CAD build for the part. Positions are in the model's coordinates, mm. Face numbers are marked on the shaded views. A direction names the side the tool comes from. Coordinates: 2 decimals unless noted, no trailing zeros. Order: outer loops, then holes, each group sorted by start corner. A loop starts at its lowest first (then second) coordinate and runs counter-clockwise, first axis right, second up. Notation, with made-up numbers: (51.5, -31.5) - (93.5, -31.5) arc R10 cw to (93.5, -22.5) - close; hole circle Ø8 at (84.5, 28). An arc over 180 degrees is marked (long way). Write each question's results on one line, items separated by ' | '. Start each with the question number.
Q1. Wall check: probe 1 along X at (y, z) = (-1.5, 19.25); probe 2 along Y at (x, z) = (-15.9, 10); probe 3 along Y at (x, z) = (-17, 12.5). Give the ranges that are in metal, low to high.
Q2. Pin check, flat tips, straight feed: P1, Ø12, axis at x = -12, z = 6.5, coming from the +Y side; P2, Ø5, axis at x = -0.63, z = 10, coming from the +Y side. Stop position of each tip, or through.
Q3. Band-saw the part on B-B, the plane y = 8. Write the cut outline in (x, z), then the cut area to 3 significant figures.
Q4. Band-saw the part on C-C, the plane z = 10. Count the separate pieces of the cut face and the enclosed holes in it, then the cut area to 3 significant figures.
Q5. Band-saw the part on D-D, the plane x = -3. Write the cut outline in (y, z), then the cut area to 3 significant figures.
Q6. Band-saw the part on A-A, the plane y = -6.5. Write the cut outline in (x, z), then the cut area to 3 significant figures.
Q7. Pull direction X, two halves, no side cores. Call the marked faces 3, 4 and 5: released by +X, released by -X, zero draft, split by the parting line, or undercut.
Q8. Which spindle directions (+Z, -Z, +X, -X, +Y, -Y) get a long thin tool onto all of the face, cutting with end or side? Do the marked faces 1 and 2. Say none if no direction does.
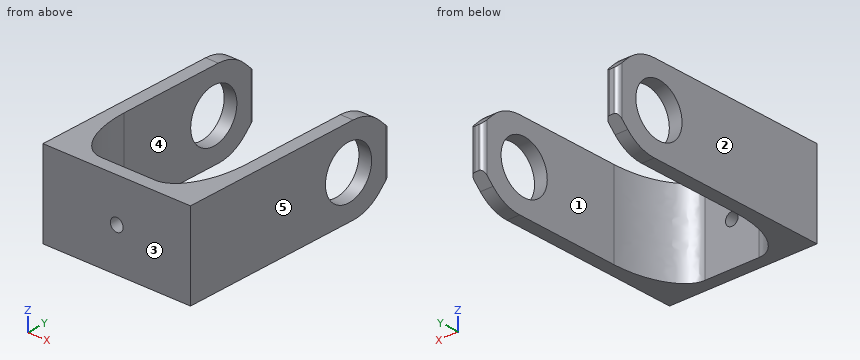
```python
from build123d import *

# Parameters (mm, degrees)
EXTRUDE_1_DEPTH     = 20
CUT_EXTRUDE_1_REACH = 52.828
SKETCH_2_R          = 6.1
SKETCH_3_R          = 1.5
CUT_EXTRUDE_2_DEPTH = 52.5
FILLET_1_R          = 10
FILLET_2_SIZE       = 15
FILLET_2_SIZE_2     = 8
FILLET_3_SIZE       = 8
FILLET_3_SIZE_2     = 15


with BuildPart() as part:
    # 草图1 → 凸台-拉伸1 (new body)
    with BuildSketch(Plane.XY):
        with BuildLine():
            Line((-18.033931645, 1.331428571), (-18.033931645, -31.183456439))
            Line((-18.033931645, -31.183456439), (16.766068355, -31.183456439))
            Line((16.766068355, -31.183456439), (16.766068355, 20.316543561))
            ThreePointArc((16.766068355, 20.316543561), (16.473175136, 21.023650343), (15.766068355, 21.316543561))
            Line((15.766068355, 21.316543561), (14.766068355, 21.316543561))
            ThreePointArc((14.766068355, 21.316543561), (14.058961574, 21.023650343), (13.766068355, 20.316543561))
            Line((13.766068355, 20.316543561), (13.766068355, -23.276677649))
            Line((13.766068355, -23.276677649), (13.766068355, -28.183456439))
            Line((13.766068355, -28.183456439), (9.089631855, -28.183456439))
            Line((9.089631855, -28.183456439), (-9.577824429, -28.183456439))
            Line((-9.577824429, -28.183456439), (-15.033931645, -28.183456439))
            Line((-15.033931645, -28.183456439), (-15.033931645, -23.510349705))
            Line((-15.033931645, -23.510349705), (-15.033931645, -10.276677649))
            Line((-15.033931645, -10.276677649), (-15.033931645, 20.316543561))
            ThreePointArc((-15.033931645, 20.316543561), (-15.326824864, 21.023650343), (-16.033931645, 21.316543561))
            Line((-16.033931645, 21.316543561), (-17.033931645, 21.316543561))
            ThreePointArc((-17.033931645, 21.316543561), (-17.741038426, 21.023650343), (-18.033931645, 20.316543561))
            Line((-18.033931645, 20.316543561), (-18.033931645, 1.331428571))
        make_face()
    extrude(amount=EXTRUDE_1_DEPTH)

    # 切除-拉伸1: up to this face of the body (flat: up to its plane)
    cut_extrude_1_end = Plane(part.part.faces().sort_by_distance((-18.033931645, -5.433456439, 10))[0])
    # 草图2 → 切除-拉伸1 (cut, up to the picked face)
    with BuildSketch(Plane(origin=(16.766068355, 0, 0), x_dir=(0, 0, -1), z_dir=(1, 0, 0)), mode=Mode.PRIVATE) as cut_extrude_1_sk1:
        with Locations((-10, 10.543673469)):
            Circle(SKETCH_2_R)
    cut_extrude_1_tool1 = split(extrude(cut_extrude_1_sk1.sketch, amount=-CUT_EXTRUDE_1_REACH, mode=Mode.PRIVATE), bisect_by=cut_extrude_1_end, keep=Keep.BOTH, mode=Mode.PRIVATE)
    # 草图2 → 切除-拉伸1 (cut, up to the picked face)
    with BuildSketch(Plane(origin=(16.766068355, 0, 0), x_dir=(0, 0, -1), z_dir=(1, 0, 0)), mode=Mode.PRIVATE) as cut_extrude_1_sk2:
        Polygon((0, 15.84743417), (-5.402663646, 21.316543561), (0, 21.316543561), align=None)
    cut_extrude_1_tool2 = split(extrude(cut_extrude_1_sk2.sketch, amount=-CUT_EXTRUDE_1_REACH, mode=Mode.PRIVATE), bisect_by=cut_extrude_1_end, keep=Keep.BOTH, mode=Mode.PRIVATE)
    # 草图2 → 切除-拉伸1 (cut, up to the picked face)
    with BuildSketch(Plane(origin=(16.766068355, 0, 0), x_dir=(0, 0, -1), z_dir=(1, 0, 0)), mode=Mode.PRIVATE) as cut_extrude_1_sk3:
        Polygon((-20, 15.84743417), (-14.597336354, 21.316543561), (-20, 21.316543561), align=None)
    cut_extrude_1_tool3 = split(extrude(cut_extrude_1_sk3.sketch, amount=-CUT_EXTRUDE_1_REACH, mode=Mode.PRIVATE), bisect_by=cut_extrude_1_end, keep=Keep.BOTH, mode=Mode.PRIVATE)
    add(cut_extrude_1_tool1.solids().sort_by(Axis((16.766068, 10.543673, 10), (-1, 0, 0)))[0], mode=Mode.SUBTRACT)
    add(cut_extrude_1_tool2.solids().sort_by(Axis((16.766068, 19.493507, 1.800888), (-1, 0, 0)))[0], mode=Mode.SUBTRACT)
    add(cut_extrude_1_tool3.solids().sort_by(Axis((16.766068, 19.493507, 18.199112), (-1, 0, 0)))[0], mode=Mode.SUBTRACT)

    # 草图3 → 切除-拉伸2 (cut)
    with BuildSketch(Plane.XZ.offset(31.183456439)):
        with Locations((-0.633931645, 10)):
            Circle(SKETCH_3_R)
    extrude(amount=-CUT_EXTRUDE_2_DEPTH, mode=Mode.SUBTRACT)

    # 圆角1
    fillet_1_edges = [part.edges().sort_by_distance(p)[0] for p in [
        (15.266068355, 15.84743417, 0),
        (15.266068355, 15.84743417, 20),
        (-16.533931645, 15.84743417, 20),
        (-16.533931645, 15.84743417, 0),
    ]]
    fillet(fillet_1_edges, radius=FILLET_1_R)

    # 圆角2
    # an asymmetric fillet: 15, 8 mm, written as the material it adds along each edge
    with BuildSketch(Plane(origin=(-15.033931645, -28.183456439, 0), x_dir=(0, 1, 0), z_dir=(0, 0, 1))) as fillet_2_piece_1:
        with BuildLine():
            Bezier((FILLET_2_SIZE, 0), (0, 0), (0, -FILLET_2_SIZE_2), weights=[1, 0.707106781, 1])
            Line((0, -FILLET_2_SIZE_2), (0, 0))
            Line((0, 0), (FILLET_2_SIZE, 0))
        make_face()
    extrude(amount=20)

    # 圆角3
    # an asymmetric fillet: 15, 8 mm, written as the material it adds along each edge
    with BuildSketch(Plane(origin=(13.766068355, -28.183456439, 0), x_dir=(-1, 0, 0), z_dir=(0, 0, 1))) as fillet_3_piece_1:
        with BuildLine():
            Bezier((FILLET_3_SIZE, 0), (0, 0), (0, -FILLET_3_SIZE_2), weights=[1, 0.707106781, 1])
            Line((0, -FILLET_3_SIZE_2), (0, 0))
            Line((0, 0), (FILLET_3_SIZE, 0))
        make_face()
    extrude(amount=20)


solid = part.part
```
Results below:
1) probe 1: x = -18.03 to -15.03, 13.77 to 16.77 | probe 2: y = -31.18 to 4.44, 16.64 to 21.31 | probe 3: y = -31.18 to 4.98, 16.11 to 21.32
2) P1: stops at y = 21.32 | P2: stops at y = -28.18
3) outline: (-18.03, 0) - (-15.03, 0) - (-15.03, 4.46) - (-18.03, 4.46) - close; (-18.03, 15.54) - (-15.03, 15.54) - (-15.03, 20) - (-18.03, 20) - close; (13.77, 0) - (16.77, 0) - (16.77, 4.46) - (13.77, 4.46) - close; (13.77, 15.54) - (16.77, 15.54) - (16.77, 20) - (13.77, 20) - close | area: 53.5 mm²
4) separate pieces: 4 | enclosed holes: 0 | area: 370 mm²
5) outline: (-31.18, 0) - (-28.18, 0) - (-28.18, 20) - (-31.18, 20) - close | area: 60.0 mm²
6) outline: (-18.03, 0) - (-15.03, 0) - (-15.03, 20) - (-18.03, 20) - close; (13.77, 0) - (16.77, 0) - (16.77, 20) - (13.77, 20) - close | area: 120 mm²
7) face 3: zero draft | face 4: undercut | face 5: released by +X
8) face 1: +Z, -Z, +Y | face 2: +Z, -Z, -X, +Y, -Y
